Work out the finished part from the listing and answer in its coordinate system (mm). A direction names the side the tool comes from. Give positions to 0.01 mm unless a question says otherwise; leave off trailing zeros. Loops run counter-clockwise (first coordinate to the right, second up) from the corner with the lowest first, then second, coordinate; pieces in that order, holes last. Notation, with made-up numbers: M 48.25,43.5 L 74.25,43.5 A25 cw 74.25,58.5 Z; hole C 20,-36 d1. An arc over 180 degrees is marked long. Write item = value, one per line. Start each with the question number.
1. The mould has two halves that part along X. Classify faces 1 (the face through (-23, -11, -104)), 2 (the face through (-16.259, -73.217, -26.622)), 3 (the face through (0, -47, -16)): released by +X, released by -X, zero draft, split by the parting line, or undercut.
2. Section C-C on z = -13 is taken. Determine the outline of the cut face in (x, y).
3. Consider L1, parallel to Y at x = 0, z = -60; L2, parallel to Z at x = -54.5, y = 17.5; L3, parallel to X at y = -15, z = -55.5. Determine where each line is inside the solid, lowest interval first. Write a range as [from, to].
4. Flat-ended cylindrical pins translate along their axes: pin 1 Ø8 at (x, z) = (48, -40.5) entering from -Y; pin 2 Ø24 at (x, y) = (1, 55.5) entering from +Z; pin 3 Ø8 at (y, z) = (23, -8) entering from -X. Find the tip coordinate at first contact, or state that the pin passes through.
5. For faces 4 (the face through (15, 1, -8)), 5 (the face through (-51, -16, -54)), 6 (the face through (-39, 1, 0)), determine the directions among +Z, -Z, +X, -X, +Y, -Y from which every point of the face is accessible in a straight line to the end or side of a thin tool.
6. Section D-D on y = 40 is taken. Determine the outline of the cut face in (x, z), plus the area to 3 significant figures.
7. Section B-B on y = 0 is taken. Determine the outline of the cut face in (x, z).
8. Section A-A on x = 0 is taken. Determine the outline of the cut face in (y, z).
Autodesk Inventor part; units mm, degrees
ref_plane "YZ Plane" through (0, 0, 0) normal (1, 0, 0) x (0, 1, 0)
ref_plane "XZ Plane" through (0, 0, 0) normal (0, 1, 0) x (-1, 0, 0)
ref_plane "XY Plane" through (0, 0, 0) normal (0, 0, 1) x (1, 0, 0)
sketch "Sketch1" plane through (0, 0, 0) normal (0, 0, 1) x (1, 0, 0)
  circle A0 centre (0, 0) radius 75
  dimension "d0" = 150
extrude "Extrusion1" add sketch "Sketch1" against normal blind 54
sketch "Sketch2" plane through (0, 0, 0) normal (0, 0, 1) x (1, 0, 0)
  line L0 (-15, 75) -> (15, 75)
  line L1 (15, 75) -> (15, -75)
  line L2 (15, -75) -> (-15, -75)
  line L3 (-15, -75) -> (-15, 75)
  point P0 (0, 0)
  dimension "d3" = 30
  dimension "d4" = 15
  dimension "d5" = 75
  dimension "d6" = 75
extrude "Extrusion2" cut sketch "Sketch2" against normal blind 16
sketch "Sketch3" plane through (0, 0, -54) normal (0, 0, -1) x (-1, 0, 0)
  circle A0 centre (0, 0) radius 53
  dimension "d9" = 106
extrude "Extrusion3" add sketch "Sketch3" along normal blind 50
sketch "Sketch4" plane through (0, 0, -104) normal (0, 0, -1) x (-1, 0, 0)
  circle A0 centre (0, 0) radius 25
  dimension "d12" = 50
extrude "Extrusion4" cut sketch "Sketch4" against normal blind 88
Verdict:
q1.face_1 = zero draft
q1.face_2 = split by the parting line
q1.face_3 = undercut
q2.outline = M -15,-73.48 L -15,73.48 A75 ccw Z; M 15,-73.48 A75 ccw 15,73.48 Z
q3.L1 = [-53, -25], [25, 53]
q3.L2 = [-54, 0]
q3.L3 = [-50.83, -20], [20, 50.83]
q4.pin_1 = -60.74
q4.pin_2 = -16
q4.pin_3 = -72.55
q5.face_4 = +Z, +Y, -Y
q5.face_5 = -Z
q5.face_6 = +Z, +X, -X, +Y, -Y
q6.outline = M -63.44,-54 L -34.77,-54 L -34.77,-104 L 34.77,-104 L 34.77,-54 L 63.44,-54 L 63.44,0 L 15,0 L 15,-16 L -15,-16 L -15,0 L -63.44,0 Z
q6.area = 9,850 mm2
q7.outline = M -75,-54 L -53,-54 L -53,-104 L -25,-104 L -25,-16 L -15,-16 L -15,0 L -75,0 Z; M 15,-16 L 25,-16 L 25,-104 L 53,-104 L 53,-54 L 75,-54 L 75,0 L 15,0 Z
q8.outline = M -75,-54 L -53,-54 L -53,-104 L -25,-104 L -25,-16 L -75,-16 Z; M 25,-104 L 53,-104 L 53,-54 L 75,-54 L 75,-16 L 25,-16 Z
